Autodesk Inventor part; units mm, degrees
ref_plane "工作平面1" through (0, 0, 0) normal (0, 0, 1) x (1, 0, 0)
ref_plane "工作平面2" through (-47.5, 0, 27) normal (0, 0, 1) x (1, 0, 0)
ref_plane "YZ Plane" through (0, 0, 0) normal (1, 0, 0) x (0, 1, 0)
ref_plane "工作平面1" through (0, 0, 0) normal (0, 0, 1) x (1, 0, 0)
sketch "草图1" plane through (0, 0, 0) normal (0, 0, 1) x (1, 0, 0)
  arc A0 (-47.5, -70) -> (-47.5, 70) centre (-47.5, 0) ccw construction
  circle A1 centre (-47.5, 0) radius 82.5 construction
  arc A2 (-47.5, -95) -> (-47.5, 95) centre (-47.5, 0) ccw construction
  line L0 (-47.5, 70) -> (-47.5, 95) construction
  arc A3 (-47.5, -70) -> (-47.5, 70) centre (-47.5, 0) ccw construction
  line L1 (-47.5, -95) -> (-47.5, -70) construction
  arc A4 (-47.5, -70) -> (-47.5, 70) centre (-47.5, 0) ccw construction
  circle A5 centre (-47.5, 0) radius 95
  circle A6 centre (-130, 0) radius 5.5
  line L2 (-180.5, 0) -> (85.5, 0) construction
  circle A7 centre (-88.75, -71.4471) radius 5.5
  circle A8 centre (-6.25, -71.4471) radius 5.5
  circle A9 centre (35, 0) radius 5.5
  circle A10 centre (-6.25, 71.4471) radius 5.5
  circle A11 centre (-88.75, 71.4471) radius 5.5
  point P0 (0, 0)
  dimension "d0" = 165
  dimension "d1" = 11
  dimension "d4" = 360
extrude "拉伸1" add sketch "草图1" along normal blind 12
sketch "草图2" plane through (-47.5, 0, 0) normal (0, 0, -1) x (-1, 0, 0)
  arc A0 (0, 70) -> (0, -70) centre (0, 0) ccw construction
  circle A1 centre (0, 0) radius 70
  circle A2 centre (0, 0) radius 60
  point P0 (-47.5, 0)
  dimension "d8" = 10
extrude "拉伸2" add sketch "草图2" along normal blind 10.5
sketch "草图3" plane through (-47.5, 0, 12) normal (0, 0, 1) x (1, 0, 0)
  circle A0 centre (0, 0) radius 70 construction
  circle A1 centre (0, 0) radius 70 construction
  circle A2 centre (0, 0) radius 72
  point P0 (47.5, 0)
  dimension "d11" = 2
ref_plane "工作平面2" through (-47.5, 0, 27) normal (0, 0, 1) x (1, 0, 0)
sketch "草图4" plane through (-47.5, 0, 27) normal (0, 0, 1) x (1, 0, 0)
  circle A0 centre (0, 0) radius 72 construction
  circle A1 centre (0, 0) radius 60
  point P0 (47.5, 0)
loft "放样1" add profiles "草图3", "草图4"
sketch "草图5" plane through (-47.5, 0, 0) normal (0, 0, -1) x (-1, 0, 0)
  circle A0 centre (0, 0) radius 60
  point P0 (-47.5, 0)
extrude "拉伸3" cut sketch "草图5" against normal blind 5
fillet "圆角1" radius 2 2 edges at (-119.5, 0, 12) (-107.5, 0, 27)
properties part number "轴承端盖2"
Here's how the part is built. I have some questions about the finished solid (model axes, mm). A direction names the side the tool comes from. Round coordinates to 2 decimals unless told otherwise and drop trailing zeros. Loops run counter-clockwise (first coordinate to the right, second up) from the corner with the lowest first, then second, coordinate; pieces in that order, holes last. Notation, with made-up numbers: (85.25, 28.25) -> (127.25, 28.25) arc R6 ccw to (127.25, 37.25) -> close; hole circle Ø5 at (76.5, 67). An arc over 180 degrees is marked (long way). Answer as CSV lines item,"result".
1. If I drill on L1, parallel to Z at x = -30, y = 15; L2, parallel to Z at x = 20.5, y = 27.5; L3, parallel to Y at x = -47, z = -9, over which ranges is the centre line in solid material (lowest first)?
Final values:
L1,"z = 5 to 27"
L2,"z = 0 to 12"
L3,"y = -70 to -60, 60 to 70"
2. Thinking about a two-plate mould opening in Y: for faces 4 (the face through (-93.115, 74.794, 5.916)), 5 (the face through (-68.09, 92.74, 5.92)), 6 (the face through (-97, 50, 0)), which applies, released by +Y, released by -Y, zero draft, split by the parting line, or undercut?
Final values:
face 4,"undercut"
face 5,"split by the parting line"
face 6,"zero draft"
3. For pin 1 (2 mm diameter, centred on y = -50.5, z = 10, fed in from -X); pin 2 (12.5 mm diameter, centred on x = -88.75, y = -71.45, fed in from -Z); pin 3 (8 mm diameter, centred on y = -44, z = 12, fed in from -X), each with a flat end and sliding along its axis, tell me the tip position at first contact or that it passes through.
Final values:
pin 1,"stops at x = -128.58"
pin 2,"stops at z = 0"
pin 3,"stops at x = -133.67"
4. If we section it at A-A on x = -47.5: Please give me the cut outline in (y, z), plus the area to 3 significant figures.
Final values:
outline,"(-95, 0) -> (-70, 0) -> (-70, -10.5) -> (-60, -10.5) -> (-60, 5) -> (60, 5) -> (60, -10.5) -> (70, -10.5) -> (70, 0) -> (95, 0) -> (95, 12) -> (72.96, 12) arc R2 cw to (71.4, 12.75) -> (60.6, 26.25) arc R2 ccw to (59.04, 27) -> (-59.04, 27) arc R2 ccw to (-60.6, 26.25) -> (-71.4, 12.75) arc R2 cw to (-72.96, 12) -> (-95, 12) -> close"
area,"3,870 mm^2"
5. If we section it at B-B on x = 35: Please give me the cut outline in (y, z).
Final values:
outline,"(-47.1, 0) -> (-5.5, 0) -> (-5.5, 12) -> (-47.1, 12) -> close; (5.5, 0) -> (47.1, 0) -> (47.1, 12) -> (5.5, 12) -> close"
6. Which directions (+Z, -Z, +X, -X, +Y, -Y) give clear straight access to the entire face, cutting with the end or side of a thin tool? Please do faces 1 (the face through (-135.495, -0.242, 5.916)), 2 (the face through (-27, 71, 12)), 3 (the face through (-47, 1, 5)).
Final values:
face 1,"+Z, -Z"
face 2,"+Z"
face 3,"-Z"
7. If we section it at C-C on z = 19: Please give me the cut outline in (x, y).
Final values:
outline,"circle Ø132.8 at (-47.5, 0)"
8. If we section it at D-D on x = -6.25: Count the separate pieces of the cut face and the enclosed holes in it, plus the area to 3 significant figures.
Final values:
separate pieces,"3"
enclosed holes,"0"
area,"3,170 mm^2"
